Autodesk Inventor part; units mm, degrees
ref_plane "YZ Plane" through (0, 0, 0) normal (1, 0, 0) x (0, 1, 0)
ref_plane "XZ Plane" through (0, 0, 0) normal (0, 1, 0) x (-1, 0, 0)
ref_plane "XY Plane" through (0, 0, 0) normal (0, 0, 1) x (1, 0, 0)
sketch "Sketch1" plane through (0, 0, 0) normal (0, 0, 1) x (1, 0, 0)
  line L0 (-28, 5) -> (28, 5)
  line L1 (28, 5) -> (28, -5)
  line L2 (28, -5) -> (-28, -5)
  line L3 (-28, -5) -> (-28, 5)
  line L4 (-10, 30) -> (10, 30)
  line L5 (10, 30) -> (10, 5)
  line L6 (10, 5) -> (-10, 5)
  line L7 (-10, 5) -> (-10, 30)
  circle A0 centre (0, 22) radius 5.15
  line L8 (-1.5, 30) -> (1.5, 30)
  line L9 (1.5, 30) -> (1.5, 8)
  line L10 (1.5, 8) -> (-1.5, 8)
  line L11 (-1.5, 8) -> (-1.5, 30)
  point P0 (0, 0)
  point P1 (-28, 0)
  point P2 (0, 5)
  point P3 (0, 30)
  point P4 (0, 30)
  point P5 (-1.5, 17.0733)
  point P6 (-1.5, 26.9267)
  point P7 (-1.5, 30)
  point P8 (-10, 5)
  point P9 (10, 5)
  point P10 (1.5, 30)
  point P11 (1.5, 26.9267)
  point P12 (1.5, 17.0733)
  dimension "d0" = 10
  dimension "d1" = 20
  dimension "d2" = 10.3
  dimension "d3" = 17
  dimension "d4" = 8
  dimension "d5" = 3
  dimension "d6" = 14
  dimension "d7" = 18
extrude "Extrusion1" add sketch "Sketch1" along normal mid plane 20 contours L0 L1 L2 L3 | L7 L4 L11 A0 L10 L9 L5 L0
sketch "Sketch2" plane through (10, 5, 10) normal (0, 1, 0) x (1, 0, 0)
  line L0 (0, 20) -> (18, 20)
  line L1 (-38, 20) -> (-20, 20)
  line L2 (-38, 20) -> (-38, 0)
  line L3 (18, 20) -> (18, 0)
  point P0 (-10, 10)
  point P1 (-30, 10)
  point P2 (10, 10)
  point P3 (-38, 10)
  point P4 (18, 10)
  dimension "d25" = 8
  dimension "d26" = 8
hole "Hole1" at (-20, 5, 0) at (20, 5, 0) direction (0, -1, 0) diameter 6 end through all
sketch "Sketch3" plane through (10, 5, 10) normal (1, 0, 0) x (0, 0, -1)
  line L0 (20, 25) -> (0, 25)
  circle A0 centre (10, 7.0733) radius 2.75
  line L1 (20, 25) -> (0, 25)
  line L2 (0, 25) -> (8, 25)
  line L3 (8, 25) -> (8, 0)
  line L4 (8, 0) -> (0, 0)
  line L5 (0, 0) -> (0, 25)
  line L6 (20, 0) -> (0, 0)
  line L7 (12, 25) -> (20, 25)
  line L8 (20, 25) -> (20, 0)
  line L9 (20, 0) -> (12, 0)
  line L10 (12, 0) -> (12, 25)
  line L11 (20, 25) -> (20, 0)
  line L12 (20, 12.0733) -> (0, 12.0733)
  point P0 (10, -5)
  point P1 (10, 25)
  point P2 (12, 0)
  dimension "d18" = 5.5
  dimension "d19" = 8
  dimension "d21" = 8
  dimension "d24" = 5
extrude "Extrusion2" cut sketch "Sketch3" against normal through all contours L10 A0 L3 | A0 L10 | L3 A0
equation "\"d21\" = d19"
properties part number "0008-10-020 Suport Axa Y"
Can you work these out from the model? Positions are in its coordinate system, mm. A direction names the side the tool comes from. Coordinates: 2 decimals unless noted, no trailing zeros. Loops run counter-clockwise (first coordinate to the right, second up) from the corner with the lowest first, then second, coordinate; pieces in that order, holes last. Notation, with made-up numbers: M -38.75,11 L -7.75,11 A26 cw -7.75,46 Z; hole C 78.25,74 d10. An arc over 180 degrees is marked long. Put each result on its own line as item: value. Start each with the question number.
(1) Imagine slicing it at D-D on z = -3.75. List the corners of the cut face in (x, y) for me.
(2) Will these pins go through, and if not, where does the flat tip stop? pin 1 Ø7 at (x, z) = (20, 0) entering from +Y; pin 2 Ø10 at (y, z) = (13.5, 5) entering from -X; pin 3 Ø3.5 at (y, z) = (12.07, 0) entering from +X; pin 4 Ø3 at (y, z) = (10, 3) entering from +X.
(3) Imagine slicing it at C-C on z = 1. Give the number of separate pieces and of enclosed holes in the cut face, and give its area (3 significant figures).
(4) Imagine slicing it at B-B on x = 20. List the corners of the cut face in (y, z) for me.
(5) Which directions (+Z, -Z, +X, -X, +Y, -Y) give clear straight access to the entire face, cutting with the end or side of a thin tool? Please do faces 1 (the face through (17, 5, 2)), 2 (the face through (-10, 17, 0)), 3 (the face through (-6, 30, 0)), 4 (the face through (0, 5, 10)), 5 (the face through (1.5, 15, -2)).
(6) Imagine slicing it at A-A on y = 15.5. List the corners of the cut face in (x, z) for me, and give its area (3 significant figures).
(7) I need wall thicknesses on probe 1 along X at (y, z) = (2, 0); probe 2 along Y at (x, z) = (-5.75, 0); probe 3 along Z at (x, y) = (20, -0.5). Which ranges of each line are inside material? Lowest first, please.
(8) We'd pull the mould along Z, two halves only. Please class faces 6 (the face through (5.81, 9.39, 0.6)), 7 (the face through (0, 5, -10)), 8 (the face through (22.93, -0.07, -0.65)), 9 (the face through (10, 18, 0)): +Z half, -Z half, draft (parallel to the pull), parting line (faces both ways), or undercut.
Worked answers:
1. outline: M -28,-5 L 28,-5 L 28,5 L 10,5 L 10,30 L 1.5,30 L 1.5,26.93 A5.15 cw 1.5,17.07 L 1.5,8 L -1.5,8 L -1.5,17.07 A5.15 cw -1.5,26.93 L -1.5,30 L -10,30 L -10,5 L -28,5 Z
2. pin 1: stops at y = 5
2. pin 2: stops at x = -10
2. pin 3: passes through
2. pin 4: stops at x = 10
3. separate pieces: 5
3. enclosed holes: 0
3. area: 741 mm2
4. outline: M -5,-10 L 5,-10 L 5,-3 L -5,-3 Z; M -5,3 L 5,3 L 5,10 L -5,10 Z
5. face 1: +Z, -Z, +X, +Y
5. face 2: +Z, -Z, -X, +Y
5. face 3: +Z, -Z, +X, -X, +Y
5. face 4: +Z, +X, -X, +Y, -Y
5. face 5: +Z, -Z, +Y
6. outline: M -10,-10 L -1.5,-10 L -1.5,10 L -10,10 Z; M 1.5,-10 L 10,-10 L 10,10 L 1.5,10 Z
6. area: 340 mm2
7. probe 1: x = -28 to -23, -17 to 17, 23 to 28
7. probe 2: y = -5 to 9.32, 14.82 to 30
7. probe 3: z = -10 to -3, 3 to 10
8. face 6: undercut
8. face 7: -Z half
8. face 8: undercut
8. face 9: draft
